Autodesk Inventor part; units mm, degrees
ref_plane "YZ Plane" through (0, 0, 0) normal (1, 0, 0) x (0, 1, 0)
ref_plane "XZ Plane" through (0, 0, 0) normal (0, 1, 0) x (-1, 0, 0)
ref_plane "XY Plane" through (0, 0, 0) normal (0, 0, 1) x (1, 0, 0)
ref_plane "Work Plane1" through (0, 0, 0) normal (0, 0, 1) x (1, 0, 0)
ref_plane "Work Plane2" through (-0.2, -170, 73.6) normal (1, 0, 0) x (0, 0, 1)
sketch "Sketch2" plane through (-0.2, -170, 73.6) normal (1, 0, 0) x (0, 0, 1)
  line L0 (-73.6, -170) -> (-73.6, 0)
  line L1 (0, 1.8) -> (-73.6, 1.8)
  line L2 (-73.6, 1.8) -> (-73.6, -103.2)
  line L3 (-73.6, -103.2) -> (0, -103.2)
  line L4 (0, -103.2) -> (0, 1.8)
  dimension "d0" = 105
extrude "Extrusion1" add sketch "Sketch2" along normal blind 3.6
sketch "Sketch3" plane through (3.4, -170, 73.6) normal (1, 0, 0) x (0, 0, -1)
  line L0 (73.6, -1.8) -> (73.6, 103.2)
  line L1 (73.6, 103.2) -> (0, 103.2)
  line L2 (0, 103.2) -> (0, -1.8)
  line L3 (0, -1.8) -> (73.6, -1.8)
  line L4 (73.6, 103.2) -> (0, 103.2) construction
  line L5 (73.6, -1.8) -> (73.6, 103.2) construction
  line L6 (36.8, 103.2) -> (73.6, 103.2) construction
  line L7 (73.6, 103.2) -> (73.6, 50.7) construction
  line L8 (73.6, 50.7) -> (36.8, 50.7) construction
  line L9 (36.8, 50.7) -> (36.8, 103.2) construction
  line L10 (16.8, 25.7) -> (56.8, 25.7)
  line L11 (61.8, 30.7) -> (61.8, 70.7)
  line L12 (56.8, 75.7) -> (16.8, 75.7)
  line L13 (11.8, 70.7) -> (11.8, 30.7)
  line L14 (11.8, 25.7) -> (61.8, 75.7) construction
  line L15 (61.8, 25.7) -> (11.8, 75.7) construction
  arc A0 (16.8, 75.7) -> (11.8, 70.7) centre (16.8, 70.7) ccw
  arc A1 (61.8, 70.7) -> (56.8, 75.7) centre (56.8, 70.7) ccw
  arc A2 (56.8, 25.7) -> (61.8, 30.7) centre (56.8, 30.7) ccw
  arc A3 (11.8, 30.7) -> (16.8, 25.7) centre (16.8, 30.7) ccw
  point P0 (73.6, 170)
  dimension "d3" = 50
  dimension "d4" = 50
  dimension "d5" = 5
extrude "Extrusion2" cut sketch "Sketch3" against normal through all contours A3 L13 A0 L12 A1 L11 A2 L10
chamfer "Chamfer1" distance 1 angle 45 4 edges at (1.6, -66.8, 73.6) (1.6, -171.8, 73.6) (1.6, -66.8, 0) (1.6, -171.8, 0)
equation "\"d1\" = wood_thickness"
properties part number "cover_components"
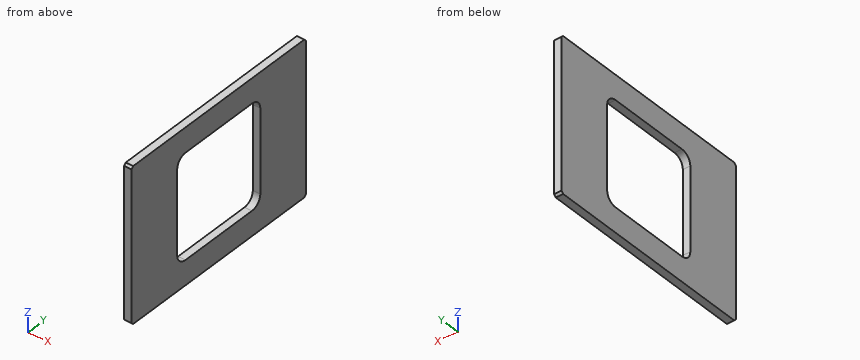
Work out the finished part from the listing and answer in its coordinate system (mm). Round coordinates to 2 decimals unless told otherwise and drop trailing zeros. Write each loop counter-clockwise with the first axis right and the second up, starting at its lowest first coordinate (ties: lowest second). Pieces come first, ordered by that corner, then holes.
1) Consider probe 1 along Y at (x, z) = (2.6, 24); probe 2 along Z at (x, y) = (1.8, -110.5); probe 3 along Z at (x, y) = (1.2, -141). Determine where each line is inside the solid, lowest interval first.
2) A cutting plane is placed at C-C on x = 0.35. Determine the outline of the cut face in (y, z), and give its area (3 significant figures).
3) A cutting plane is placed at B-B on z = 53.5. Determine the outline of the cut face in (x, y).
4) A cutting plane is placed at A-A on y = -136.5. Determine the outline of the cut face in (x, z), and give its area (3 significant figures).
Entries:
1. probe 1: y = -171.8 to -144.3, -94.3 to -66.8
1. probe 2: z = 0 to 11.8, 61.8 to 73.6
1. probe 3: z = 0 to 12.1, 61.5 to 73.6
2. outline: (-171.8, 1) - (-170.8, 0) - (-67.8, 0) - (-66.8, 1) - (-66.8, 72.6) - (-67.8, 73.6) - (-170.8, 73.6) - (-171.8, 72.6) - close; hole (-144.3, 16.8) arc R5 ccw to (-139.3, 11.8) - (-99.3, 11.8) arc R5 ccw to (-94.3, 16.8) - (-94.3, 56.8) arc R5 ccw to (-99.3, 61.8) - (-139.3, 61.8) arc R5 ccw to (-144.3, 56.8) - close
2. area: 5,250 mm2
3. outline: (-0.2, -171.8) - (3.4, -171.8) - (3.4, -144.3) - (-0.2, -144.3) - close; (-0.2, -94.3) - (3.4, -94.3) - (3.4, -66.8) - (-0.2, -66.8) - close
4. outline: (-0.2, 0) - (3.4, 0) - (3.4, 11.8) - (-0.2, 11.8) - close; (-0.2, 61.8) - (3.4, 61.8) - (3.4, 73.6) - (-0.2, 73.6) - close
4. area: 85.0 mm2
